from build123d import *
from OCP.BRepFilletAPI import BRepFilletAPI_MakeChamfer

# Parameters (mm, degrees)
ESQUISSE1_R             = 16
BASE_EXTRUSION_DEPTH    = 8.5
CHANFREIN1_SIZE         = 2.5
CHANFREIN1_SIZE2        = 1.443375673
ESQUISSE2_OUTSIDE_W     = 43.21
ESQUISSE2_OUTSIDE_H     = 43.21
ENL_V_MAT_EXTRU_1_DEPTH = 25.171263931
ESQUISSE3_R             = 13.5
BOSS_EXTRU_1_DEPTH      = 0.5
ESQUISSE4_R             = 10.5
BOSS_EXTRU_2_DEPTH      = 13
CHANFREIN2_SIZE         = 1
CHANFREIN2_SIZE2        = 1.732050808
ESQUISSE5_OUTSIDE_W     = 38.348
ESQUISSE5_OUTSIDE_H     = 42.524
ESQUISSE5_OUTSIDE_R     = 8.75
ENL_V_MAT_EXTRU_2_DEPTH = 3
CONG_1_R                = 1.5


with BuildPart() as part:
    # Esquisse1 → Base-Extrusion (new body)
    with BuildSketch(Plane.XY):
        Circle(ESQUISSE1_R)
    extrude(amount=BASE_EXTRUSION_DEPTH)

    # Chanfrein1: one chamfer whose edges measure the first distance from different faces: ONE call of the kernel's chamfer builder (chamfer() names one face for all edges)
    chanfrein1_edges_1 = [part.edges().sort_by_distance(p)[0] for p in [
        (-16, 0, 0),
    ]]
    chanfrein1_side_1 = [part.faces().sort_by_distance(p)[0] for p in [
        (0, 0, 0),
    ]]
    chanfrein1_edges_2 = [part.edges().sort_by_distance(p)[0] for p in [
        (-16, 0, 8.5),
    ]]
    chanfrein1_side_2 = [part.faces().sort_by_distance(p)[0] for p in [
        (0, 0, 8.5),
    ]]
    chanfrein1 = BRepFilletAPI_MakeChamfer(part.part.solid().wrapped)
    for e in chanfrein1_edges_1:
        chanfrein1.Add(CHANFREIN1_SIZE, CHANFREIN1_SIZE2, e.wrapped, chanfrein1_side_1[0].wrapped)  # the first distance lies on this face
    for e in chanfrein1_edges_2:
        chanfrein1.Add(CHANFREIN1_SIZE, CHANFREIN1_SIZE2, e.wrapped, chanfrein1_side_2[0].wrapped)  # the first distance lies on this face
    add(Compound.cast(chanfrein1.Shape()), mode=Mode.REPLACE)

    # Esquisse2 outside → Enlèv. mat.-Extru.1 (cut, through all)
    with BuildSketch(Plane.XY.offset(8.5)):
        Rectangle(ESQUISSE2_OUTSIDE_W, ESQUISSE2_OUTSIDE_H)
        Polygon((13.5, -7.794228634), (13.5, 7.794228634), (0, 15.588457268), (-13.5, 7.794228634), (-13.5, -7.794228634), (0, -15.588457268), align=None, mode=Mode.SUBTRACT)
    extrude(amount=-ENL_V_MAT_EXTRU_1_DEPTH, mode=Mode.SUBTRACT)

    # Esquisse3 → Boss.-Extru.1 (add)
    with BuildSketch(Plane.XY.offset(8.5)):
        Circle(ESQUISSE3_R)
    extrude(amount=BOSS_EXTRU_1_DEPTH)

    # Esquisse4 → Boss.-Extru.2 (add)
    with BuildSketch(Plane.XY.offset(9)):
        with Locations(Location((0, 0, 0), (0, 0, 180))):
            Circle(ESQUISSE4_R)
    extrude(amount=BOSS_EXTRU_2_DEPTH)

    # Chanfrein2
    chanfrein2_edges = [part.edges().sort_by_distance(p)[0] for p in [
        (10.5, 0, 22),
    ]]
    chanfrein2_side = [part.faces().sort_by_distance(p)[0] for p in [
        (10.5, 0, 15.5),
    ]]
    chamfer(chanfrein2_edges, length=CHANFREIN2_SIZE, length2=CHANFREIN2_SIZE2, reference=chanfrein2_side[0])

    # Esquisse5 outside → Enlèv. mat.-Extru.2 (cut)
    with BuildSketch(Plane.XY.offset(9)):
        Rectangle(ESQUISSE5_OUTSIDE_W, ESQUISSE5_OUTSIDE_H)
        Circle(ESQUISSE5_OUTSIDE_R, mode=Mode.SUBTRACT)
    extrude(amount=ENL_V_MAT_EXTRU_2_DEPTH, mode=Mode.SUBTRACT)

    # Congé1
    cong_1_edges = [part.edges().sort_by_distance(p)[0] for p in [
        (-8.75, 0, 9),
        (-8.75, 0, 12),
    ]]
    fillet(cong_1_edges, radius=CONG_1_R - 0.0001)  # a hair under: the kernel refuses the full size


solid = part.part
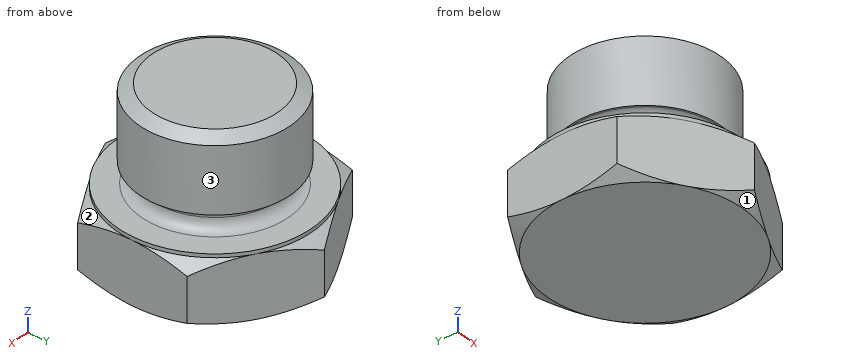
Can you work these out from the model? Positions are in its coordinate system, mm. Face numbers are marked on the shaded views. Round coordinates to 2 decimals unless told otherwise and drop trailing zeros. Loops run counter-clockwise (first coordinate to the right, second up) from the corner with the lowest first, then second, coordinate; pieces in that order, holes last. Notation, with made-up numbers: (76.5, 36) - (96.5, 36) arc R28 ccw to (96.5, 65) - close; hole circle Ø7 at (-33, 79). An arc over 180 degrees is marked (long way). Answer in a Markdown table with one row per item. Add a question column.
Q1. I need wall thicknesses on L1, parallel to Z at x = -3.75, y = 11.5; L2, parallel to Y at x = -9.25, z = 3; L3, parallel to Y at x = -0.25, z = 8. Which ranges of each line are inside material? Lowest first, please.
Q2. I want a section at A-A on z = 5.5. List the corners of the cut face in (x, y) for me, and give its area (3 significant figures).
Q3. I want a section at C-C on z = 11.25. List the corners of the cut face in (x, y) for me, and give its area (3 significant figures).
Q4. We'd pull the mould along Z, two halves only. Please class the marked faces 1, 2 and 3: pulls with the +Z half, pulls with the -Z half, needs draft (parallel to the pull), parting line crosses it, or undercut.
Q5. For pin 1 Ø1 at (x, z) = (-4, 14.5) entering from -Y; pin 2 Ø1.5 at (y, z) = (-3.5, 13.5) entering from -X; pin 3 Ø12 at (x, z) = (-9.5, 8) entering from +Y; pin 4 Ø6 at (x, y) = (-4.5, -6) entering from -Z, each with a flat end and sliding along its axis, tell me the tip position at first contact or that it passes through.
Q6. I want a section at B-B on z = 17. List the corners of the cut face in (x, y) for me, and give its area (3 significant figures).
A:
| question | item | result |
|---|---|---|
| 1 | L1 | 0 to 9 |
| 1 | L2 | -10.25 to 10.25 |
| 1 | L3 | -14.36 to 14.36 |
| 2 | outline | (-13.5, -7.79) - (0, -15.59) - (13.5, -7.79) - (13.5, 7.79) - (0, 15.59) - (-13.5, 7.79) - close |
| 2 | area | 631 mm^2 |
| 3 | outline | circle Ø17.9 at (0, 0) |
| 3 | area | 252 mm^2 |
| 4 | face 1 | pulls with the -Z half |
| 4 | face 2 | pulls with the +Z half |
| 4 | face 3 | needs draft |
| 5 | pin 1 | y = -9.9 |
| 5 | pin 2 | x = -10.13 |
| 5 | pin 3 | y = 13.57 |
| 5 | pin 4 | z = 0 |
| 6 | outline | circle Ø21 at (0, 0) |
| 6 | area | 346 mm^2 |
